Could you check a few things on this drawing? It's one solid part, dimensions in mm from its lowest x, y, z. A direction names the side the tool comes from. Give positions to 0.01 mm unless a question says otherwise; leave off trailing zeros. Write each loop counter-clockwise with the first axis right and the second up, starting at its lowest first coordinate (ties: lowest second). Pieces come first, ordered by that corner, then holes. Notation, with made-up numbers: (-6.75, 89) -> (2.25, 89) arc R23 ccw to (2.25, 102) -> close; hole circle Ø2 at (74, -33). An arc over 180 degrees is marked (long way). Answer as CSV lines item,"result". Start each with the question number.
1. On a 3-axis mill with a long thin cutter (end or side, diameter ignored), from which of +Z, -Z, +X, -X, +Y, -Y can I reach the whole of each face in a straight line? I mean the marked faces 4 and 5. Say none if no direction works.
2. If we section it at C-C on y = 9.25: Write out the boundary of the cut face in (x, z), plus the area to 3 significant figures.
3. If we section it at A-A on z = 16.75: Write out the boundary of the cut face in (x, y), plus the area to 3 significant figures.
4. I'm going to push flat-ended pins straight in: P1, Ø4.5, axis at x = 4.5, y = 9.5, coming from the +Z side; P2, Ø1, axis at y = 13, z = 13, coming from the +X side. Where does each tip first touch, or does it pass through?
5. If we mould it in two halves opening along Y, with no side actions, what happens to the marked faces 1, 2 and 3? For each: pulls with the +Y half, pulls with the -Y half, needs draft (parallel to the pull), parting line crosses it, or undercut.
6. If we section it at B-B on x = 2.75: Write out the boundary of the cut face in (y, z).
7. I need wall thicknesses on line 1 (Y direction, x = 8.5, z = 13); line 2 (Z direction, x = 7, y = 4.5). Which ranges of each line are inside material? Lowest first, please. Write a range as [from, to].
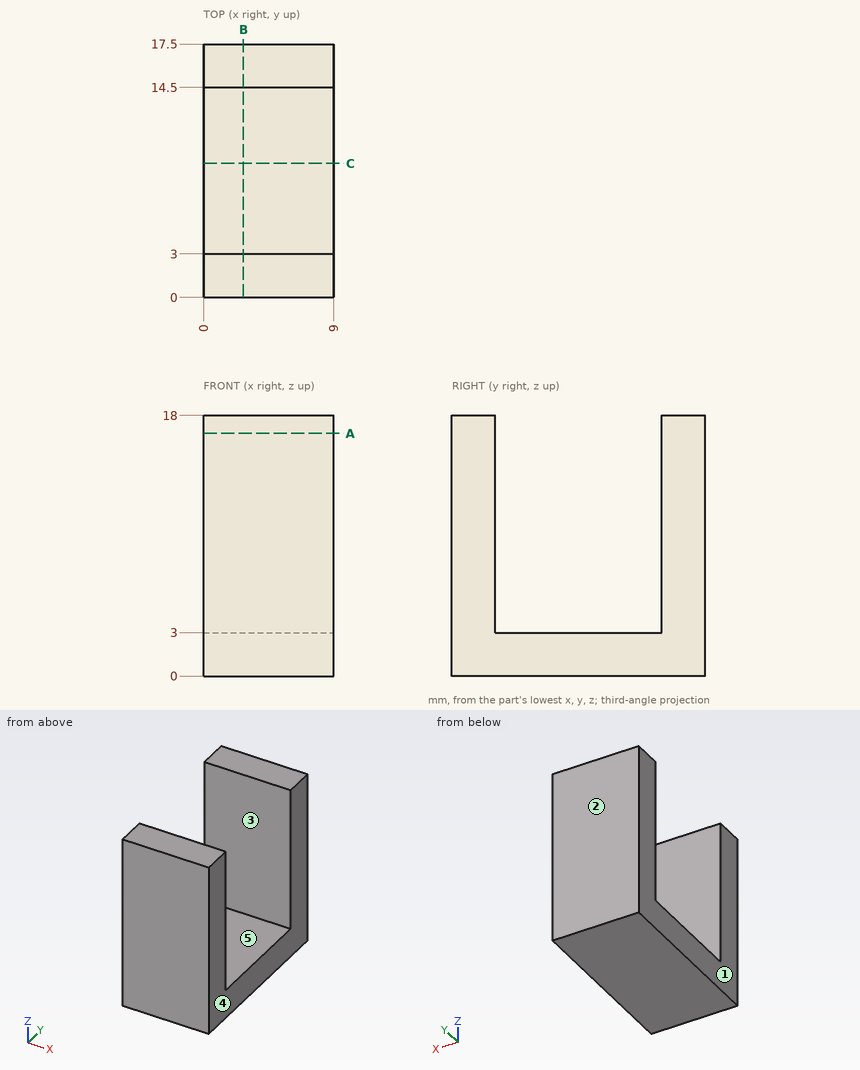
Computed values:
1,face 4,"+Z, -Z, +X, +Y, -Y"
1,face 5,"+Z, +X, -X"
2,outline,"(0, 0) -> (9, 0) -> (9, 3) -> (0, 3) -> close"
2,area,"27.0 mm2"
3,outline,"(0, 0) -> (9, 0) -> (9, 3) -> (0, 3) -> close; (0, 14.5) -> (9, 14.5) -> (9, 17.5) -> (0, 17.5) -> close"
3,area,"54.0 mm2"
4,P1,"stops at z = 3"
4,P2,"passes through"
5,face 1,"needs draft"
5,face 2,"pulls with the +Y half"
5,face 3,"undercut"
6,outline,"(0, 0) -> (17.5, 0) -> (17.5, 18) -> (14.5, 18) -> (14.5, 3) -> (3, 3) -> (3, 18) -> (0, 18) -> close"
7,line 1,"y = [0, 3], [14.5, 17.5]"
7,line 2,"z = [0, 3]"
